```python
from build123d import *

# Parameters (mm, degrees)
SKETCH1_R               = 4.7625
BOSS_EXTRUDE1_DEPTH     = 5.08
SKETCH4_W               = 19.05
SKETCH4_H               = 5.08
BOSS_EXTRUDE2_DEPTH     = 5.08
SKETCH5_R               = 1.651
SKETCH5_R_2             = 1.660728382
CUT_EXTRUDE1_DEPTH      = 1.0000001
CUT_EXTRUDE1_DEPTH_BACK = 6.0800001
SKETCH6_R               = 4.7625
BOSS_EXTRUDE3_DEPTH     = 5.08
SKETCH8_R               = 4.7625
CUT_EXTRUDE2_DEPTH      = 6.0800001


with BuildPart() as part:
    # Sketch1 → Boss-Extrude1 (new body)
    with BuildSketch(Plane(origin=(0, 0, 0), x_dir=(1, 0, 0), z_dir=(0, 1, 0))):
        with BuildLine():
            Line((-9.525, 53.975), (9.525, 53.975))
            Line((9.525, 53.975), (9.525, 51.435))
            add(Edge.make_bspline(
                [(9.525, 51.435), (9.525, 51.21454564), (27.819109584, -48.895), (60.325, -48.895)],
                knots=[0, 0, 0, 0, 1, 1, 1, 1], degree=3))
            Line((60.325, -48.895), (-9.525, -48.895))
            Line((-9.525, -48.895), (-9.525, 53.975))
        make_face()
        with Locations((0, 45.9867)):
            Circle(SKETCH1_R, mode=Mode.SUBTRACT)
    extrude(amount=BOSS_EXTRUDE1_DEPTH)

    # Sketch4 → Boss-Extrude2 (add)
    with BuildSketch(Plane(origin=(0, 5.08, 0), x_dir=(1, 0, 0), z_dir=(0, 1, 0))):
        with Locations((50.8, -51.435)):
            Rectangle(SKETCH4_W, SKETCH4_H)
    extrude(amount=-BOSS_EXTRUDE2_DEPTH)

    # Sketch5 → Cut-Extrude1 (cut, two sides)
    with BuildSketch(Plane.XZ) as cut_extrude1_sk:
        with Locations((34.925, 40.005)):
            Circle(SKETCH5_R)
        with Locations((-3.175, 4.445)):
            Circle(SKETCH5_R_2)
    extrude(amount=CUT_EXTRUDE1_DEPTH, mode=Mode.SUBTRACT)
    extrude(cut_extrude1_sk.sketch, amount=-CUT_EXTRUDE1_DEPTH_BACK, mode=Mode.SUBTRACT)

    # Sketch6 → Boss-Extrude3 (add)
    with BuildSketch(Plane.XZ):
        with BuildLine():
            Line((-13.589, -18.81432439), (-9.525, -18.81432439))
            Line((-9.525, -18.81432439), (-9.525, -19.686347414))
            ThreePointArc((-9.525, -19.686347414), (-3.683, -28.72032439), (-9.525, -37.754301365))
            Line((-9.525, -37.754301365), (-9.525, -38.62632439))
            Line((-9.525, -38.62632439), (-13.589, -38.62632439))
            ThreePointArc((-13.589, -38.62632439), (-23.495, -28.72032439), (-13.589, -18.81432439))
        make_face()
        with Locations((-13.589, -28.72032439)):
            Circle(SKETCH6_R, mode=Mode.SUBTRACT)
    extrude(amount=-BOSS_EXTRUDE3_DEPTH)

    # Sketch8 → Cut-Extrude2 (cut, through all)
    with BuildSketch(Plane(origin=(0, 5.08, 0), x_dir=(1, 0, 0), z_dir=(0, 1, 0))):
        with Locations((-13.589, 28.72032439)):
            Circle(SKETCH8_R)
    extrude(amount=-CUT_EXTRUDE2_DEPTH, mode=Mode.SUBTRACT)


solid = part.part
```
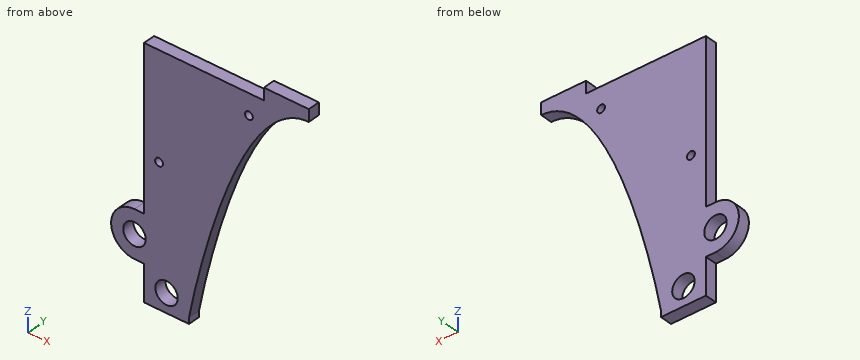
The listing builds one solid part. Answer for the finished solid, in the listing's coordinates (mm). Give positions to 0.01 mm unless a question says otherwise; leave off trailing zeros. Loops run counter-clockwise (first coordinate to the right, second up) from the corner with the lowest first, then second, coordinate; pieces in that order, holes last. Notation, with made-up numbers: (20, 5.25) - (57, 5.25) arc R11 cw to (57, 12.25) - close; hole circle Ø8 at (67, 30.5). An arc over 180 degrees is marked (long way). Return JSON: item names as keys, results as strings. Group by question number.
1. Find section B-B (y = 1.3). State how many separate pieces and enclosed holes the cut face has, then the cut area to 3 significant figures.
2. Straight lines are drawn through the part: line 1 (Z direction, x = 0, y = 2.45) (3 decimals); line 2 (Z direction, x = 2, y = 1.7) (1 decimal); line 3 (Z direction, x = -3, y = 0.25) (3 decimals). For each, find the intervals that lie inside material, in ascending order. Write a range as [from, to].
3. Given pin 1 Ø1.5 at (x, y) = (33.5, 0.5) entering from +Z (3 decimals); pin 2 Ø2 at (y, z) = (3.5, 28) entering from +X; pin 3 Ø1.5 at (y, z) = (3, -47.5) entering from -X (3 decimals); pin 4 Ø5.5 at (x, z) = (-13.59, -28.72) entering from +Y, each flat-ended and moving along its own axis, determine where each tip first touches the part or whether it passes through.
4. Find section A-A (x = 0). Write down the section's boundary in (y, z) (3 decimals).
Verdict:
{
 "1": {"separate pieces": "1", "enclosed holes": "4", "area": "3,700 mm^2"},
 "2": {"line 1": "z = [-53.975, -50.749], [-41.224, 48.895]", "line 2": "z = [-54, -50.3], [-41.7, 48.9]", "line 3": "z = [-53.975, -49.686], [-42.288, 2.794], [6.096, 48.895]"},
 "3": {"pin 1": "stops at z = 48.895", "pin 2": "stops at x = 36.01", "pin 3": "stops at x = -9.525", "pin 4": "passes through"},
 "4": {"outline": "(0, -53.975) - (5.08, -53.975) - (5.08, -50.749) - (0, -50.749) - close; (0, -41.224) - (5.08, -41.224) - (5.08, 48.895) - (0, 48.895) - close"}
}
